Read the model definition and answer for the solid it produces. Units are mm, in the model's axes. Face numbers are marked on the shaded views. Coordinates: 2 decimals unless noted, no trailing zeros. Loops run counter-clockwise (first coordinate to the right, second up) from the corner with the lowest first, then second, coordinate; pieces in that order, holes last. Notation, with made-up numbers: M -14,-29 L 31,-29 A24 cw 31,-5 Z; hole C -2.75,22.25 d1. An arc over 180 degrees is marked long. One line per item, written item: value. Start each with the question number.
1. Determine the mould class of the marked faces 1, 2, 3 and 4 for opening direction X: +X half, -X half, draft (parallel to the pull), parting line (faces both ways), or undercut.
2. The part is cut by section B-B (y = 12.7). Write down the section's boundary in (x, z).
3. The part is cut by section C-C (y = 319). Write down the section's boundary in (x, z) (3 decimals), then the cut area to 3 significant figures.
4. Flat-ended cylindrical pins translate along their axes: pin 1 (1 mm diameter, centred on x = 66, y = 478.5, fed in from +Z); pin 2 (7.5 mm diameter, centred on x = 119.6, y = 12.7, fed in from +Z). Find the tip coordinate at first contact, or state that the pin passes through.
5. Consider probe 1 along Z at (x, y) = (74.5, 563); probe 2 along Y at (x, z) = (20, 39). Determine where each line is inside the solid, lowest interval first.
6. The part is cut by section A-A (x = 25.4). Write down the section's boundary in (y, z) (3 decimals).
```python
from build123d import *

# Parameters (mm, degrees)
F0_W     = 144.999558
F0_H     = 599.998292
F1_DEPTH = 44.999859
F2_W     = 138.649558
F2_H     = 568.248292
F3_DEPTH = 1.27
F4_R     = 6.35
F5_DEPTH = 12.7


with BuildPart() as f1:
    # F0 (on Top) → F1 (new body)
    with BuildSketch(Plane.XY):
        with Locations((72.499779, 299.999146)):
            Rectangle(F0_W, F0_H)
    extrude(amount=F1_DEPTH)

    # F2 (on face) → F3 (cut)
    with BuildSketch(Plane.XY.offset(44.999859)):
        with Locations((72.499779, 312.699146)):
            Rectangle(F2_W, F2_H)
    extrude(amount=-F3_DEPTH, mode=Mode.SUBTRACT)

    # F4 (on face) → F5 (cut)
    with BuildSketch(Plane.XY.offset(44.999859)):
        with Locations((25.4, 12.7)):
            Circle(F4_R)
        with Locations((119.599558, 12.7)):
            Circle(F4_R)
    extrude(amount=-F5_DEPTH, mode=Mode.SUBTRACT)


solid = f1.part
```
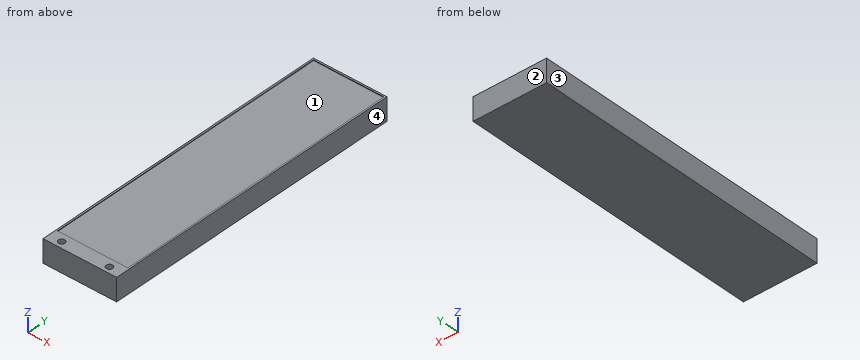
Answer block:
1. face 1: undercut
1. face 2: draft
1. face 3: -X half
1. face 4: +X half
2. outline: M 0,0 L 145,0 L 145,45 L 125.95,45 L 125.95,32.3 L 113.25,32.3 L 113.25,45 L 31.75,45 L 31.75,32.3 L 19.05,32.3 L 19.05,45 L 0,45 Z
3. outline: M 0,0 L 145,0 L 145,45 L 141.825,45 L 141.825,43.73 L 3.175,43.73 L 3.175,45 L 0,45 Z
3. area: 6,350 mm2
4. pin 1: stops at z = 43.73
4. pin 2: stops at z = 32.3
5. probe 1: z = 0 to 43.73
5. probe 2: y = 0 to 9.36, 16.04 to 600
6. outline: M 0,0 L 599.998,0 L 599.998,45 L 596.823,45 L 596.823,43.73 L 28.575,43.73 L 28.575,45 L 19.05,45 L 19.05,32.3 L 6.35,32.3 L 6.35,45 L 0,45 Z
